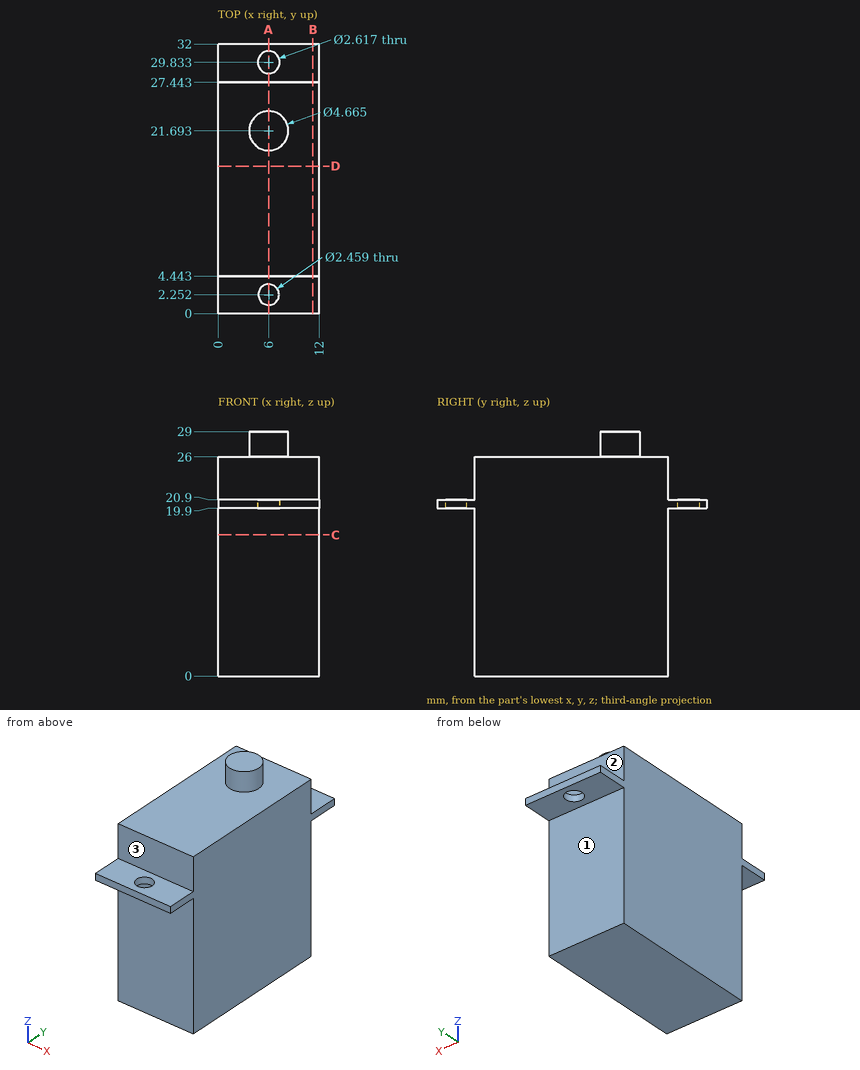
Could you check a few things on this drawing? It's one solid part, dimensions in mm from its lowest x, y, z. A direction names the side the tool comes from. Give positions to 0.01 mm unless a question says otherwise; leave off trailing zeros. Order: outer loops, then holes, each group sorted by start corner. A loop starts at its lowest first (then second) coordinate and runs counter-clockwise, first axis right, second up.
1. For pin 1 (2.5 mm diameter, centred on x = 3, z = 22.5, fed in from +Y); pin 2 (1 mm diameter, centred on x = 6.5, z = 8, fed in from -Y); pin 3 (2.5 mm diameter, centred on x = 5, y = 30, fed in from +Z), each with a flat end and sliding along its axis, tell me the tip position at first contact or that it passes through.
Answers below:
pin 1: stops at y = 27.44
pin 2: stops at y = 4.44
pin 3: stops at z = 20.9
2. Which directions (+Z, -Z, +X, -X, +Y, -Y) give clear straight access to the entire face, cutting with the end or side of a thin tool? Please do the marked faces 1, 2 and 3.
Answers below:
face 1: -Z, +X, -X, +Y
face 2: +Z, +X, -X, +Y
face 3: +Z, +X, -X, -Y
3. Suppose I cut it at C-C (z = 16.75). Write out the boundary of the cut face in (x, y).
Answers below:
outline: (0, 4.44) - (12, 4.44) - (12, 27.44) - (0, 27.44) - close
4. I need wall thicknesses on L1, parallel to Y at x = 6, z = 20.35 (1 decimal); L2, parallel to Z at x = 6.75, y = 15.5; L3, parallel to Y at x = 1, z = 9. Which ranges of each line are inside material? Lowest first, please.
Answers below:
L1: y = 0 to 1, 3.5 to 28.5, 31.1 to 32
L2: z = 0 to 26
L3: y = 4.44 to 27.44
5. Suppose I cut it at B-B (x = 11.25). Write out the boundary of the cut face in (y, z).
Answers below:
outline: (0, 19.9) - (4.44, 19.9) - (4.44, 0) - (27.44, 0) - (27.44, 19.9) - (32, 19.9) - (32, 20.9) - (27.44, 20.9) - (27.44, 26) - (4.44, 26) - (4.44, 20.9) - (0, 20.9) - close
6. Suppose I cut it at A-A (x = 6). Write out the boundary of the cut face in (y, z) (1 decimal).
Answers below:
outline: (0, 19.9) - (1, 19.9) - (1, 20.9) - (0, 20.9) - close; (3.5, 19.9) - (4.4, 19.9) - (4.4, 0) - (27.4, 0) - (27.4, 19.9) - (28.5, 19.9) - (28.5, 20.9) - (27.4, 20.9) - (27.4, 26) - (24, 26) - (24, 29) - (19.4, 29) - (19.4, 26) - (4.4, 26) - (4.4, 20.9) - (3.5, 20.9) - close; (31.1, 19.9) - (32, 19.9) - (32, 20.9) - (31.1, 20.9) - close
7. Suppose I cut it at D-D (y = 17.5). Write out the boundary of the cut face in (x, z), plus the area to 3 significant figures.
Answers below:
outline: (0, 0) - (12, 0) - (12, 26) - (0, 26) - close
area: 312 mm2
